Drawing for the job (mm, zero at the part's lowest x, y, z). Give positions to 0.01 mm unless a question says otherwise; leave off trailing zeros. Loops run counter-clockwise (first coordinate to the right, second up) from the corner with the lowest first, then second, coordinate; pieces in that order, holes last. Notation, with made-up numbers: M -40,-15 L 17,-15 A21 cw 17,2 Z; hole C 84.25,-35 d9. An arc over 180 degrees is marked long. Use CSV: the item, a comma, the result in double quotes. Start each with the question number.
(1) Wall check: line 1 along Z through (x, y) = (122, 3.8); line 2 along Z through (x, y) = (122, 1.35); line 3 along Z through (x, y) = (112, 3.6). Give the ranges that are in metal, low to high. Write a range as from..to.
(2) Slice it at A-A on z = 25. List the corners of the cut face in (x, y), and give its area (3 significant figures).
(3) Slice it at B-B on x = 88. List the corners of the cut face in (y, z), and give its area (3 significant figures).
(4) Flat gauge pin, fed straight in: P1, Ø5.5, axis at x = 78, z = 122, coming from the -Y side. Where does the tip first touch, or does it go through?
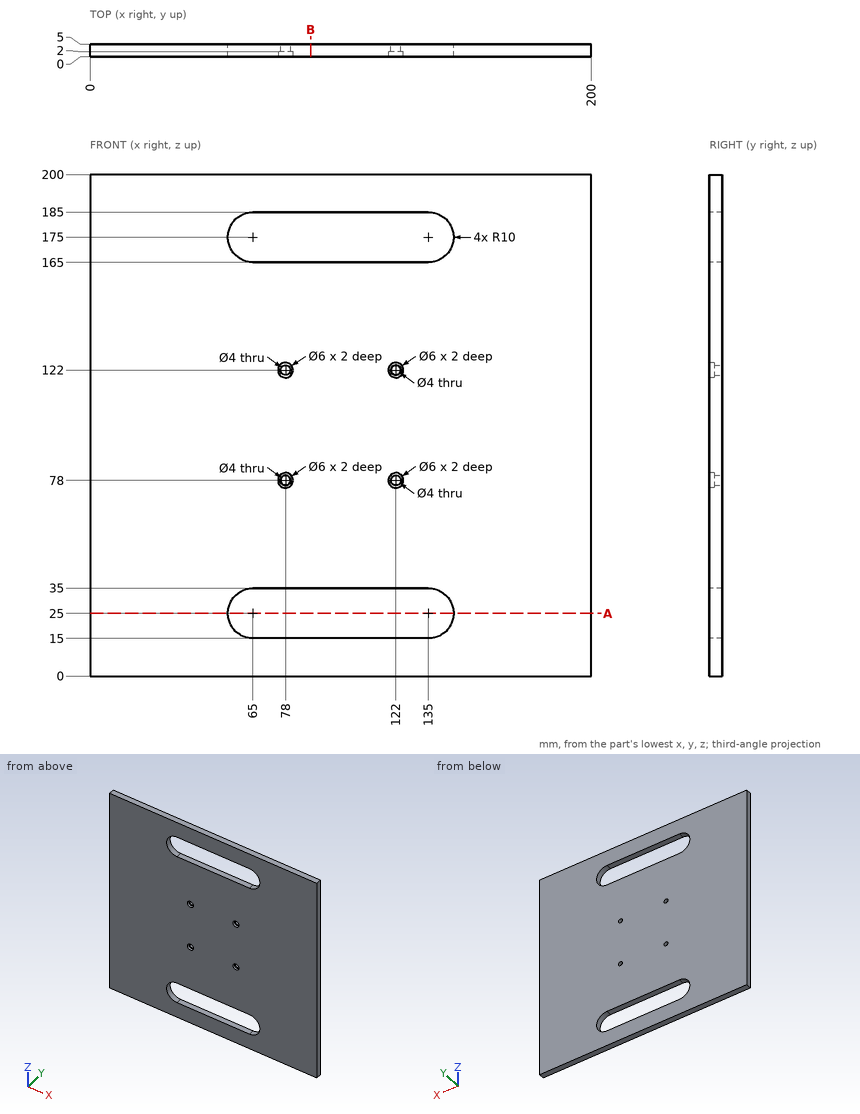
Reply:
1,line 1,"z = 0..15, 35..76, 80..120, 124..165, 185..200"
1,line 2,"z = 0..15, 35..75, 81..119, 125..165, 185..200"
1,line 3,"z = 0..15, 35..165, 185..200"
2,outline,"M 0,0 L 55,0 L 55,5 L 0,5 Z; M 145,0 L 200,0 L 200,5 L 145,5 Z"
2,area,"550 mm^2"
3,outline,"M 0,0 L 5,0 L 5,15 L 0,15 Z; M 0,35 L 5,35 L 5,165 L 0,165 Z; M 0,185 L 5,185 L 5,200 L 0,200 Z"
3,area,"800 mm^2"
4,P1,"stops at y = 2"
